```python
from build123d import *

# Parameters (mm, degrees)
BOSS_EXTRUDE4_DEPTH = 20
SKETCH6_R           = 1.75
CUT_EXTRUDE3_DEPTH  = 51.482948977
SKETCH7_R           = 3.3782
CUT_EXTRUDE4_DEPTH  = 52.051285634
SKETCH8_W           = 5.5
SKETCH8_H           = 5
BOSS_EXTRUDE5_DEPTH = 5


with BuildPart() as part:
    # Sketch5 → Boss-Extrude4 (new body)
    with BuildSketch(Plane(origin=(0, 0, 0), x_dir=(0, 0, -1), z_dir=(1, 0, 0))):
        Polygon((0, 0), (0, 20), (-21.213203436, 41.213203436), (-25.213203436, 41.213203436), (-4, 20), (-4, 0), align=None)
    extrude(amount=BOSS_EXTRUDE4_DEPTH)

    # Sketch6 → Cut-Extrude3 (cut, through all)
    with BuildSketch(Plane.XY.offset(4)):
        with Locations((10, 10)):
            Circle(SKETCH6_R)
    extrude(amount=-CUT_EXTRUDE3_DEPTH, mode=Mode.SUBTRACT)

    # Sketch7 → Cut-Extrude4 (cut, through all)
    with BuildSketch(Plane(origin=(0, 8, -8), x_dir=(1, 0, 0), z_dir=(0, -0.7071067811865489, 0.7071067811865462))):
        with Locations(Location((10, 31.970562748, 0), (0, 0, 270))):
            Circle(SKETCH7_R)
    extrude(amount=-CUT_EXTRUDE4_DEPTH, mode=Mode.SUBTRACT)

    # Sketch8 → Boss-Extrude5 (add)
    with BuildSketch(Plane(origin=(0, 0, 0), x_dir=(-1, 0, 0), z_dir=(0, 0, -1))):
        with Locations((-10, 17.5)):
            Rectangle(SKETCH8_W, SKETCH8_H)
        with Locations((-10, 2.5)):
            Rectangle(SKETCH8_W, SKETCH8_H)
    extrude(amount=BOSS_EXTRUDE5_DEPTH)


solid = part.part
```
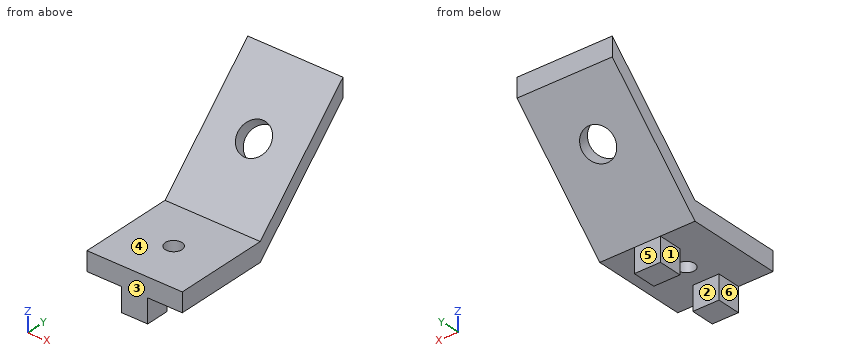
Geometry check sheet. Reference: the model listing, model coordinates, mm. Face numbers are marked on the shaded views. A direction names the side the tool comes from. Coordinates: 2 decimals unless noted, no trailing zeros. Order: outer loops, then holes, each group sorted by start corner. A loop starts at its lowest first (then second) coordinate and runs counter-clockwise, first axis right, second up.
Q1. Sectioned sample at B-B on x = 10. Record the cut outline in (y, z).
Reply:
outline: (0, -5) - (5, -5) - (5, 0) - (8.25, 0) - (8.25, 4) - (0, 4) - close; (11.75, 0) - (15, 0) - (15, -5) - (20, -5) - (20, 0) - (30.22, 10.22) - (28.22, 12.22) - (20, 4) - (11.75, 4) - close; (33, 17) - (35, 15) - (41.21, 21.21) - (41.21, 25.21) - close
Q2. Thickness scan on probe 1 along Y at (x, z) = (10, 1.1); probe 2 along Y at (x, z) = (10, 2.4); probe 3 along Z at (x, y) = (16.5, 12). Record the ranges inside material, lowest first.
Reply:
probe 1: y = 0 to 8.25, 11.75 to 21.1
probe 2: y = 0 to 8.25, 11.75 to 22.4
probe 3: z = 0 to 4
Q3. Sectioned sample at A-A on y = 10. Record the cut outline in (x, z).
Reply:
outline: (0, 0) - (8.25, 0) - (8.25, 4) - (0, 4) - close; (11.75, 0) - (20, 0) - (20, 4) - (11.75, 4) - close
Q4. Depth check by flat-ended pin: pin 1 Ø3 at (x, z) = (14, 15) entering from +Y; pin 2 Ø1 at (x, z) = (5, 13.5) entering from +Y; pin 3 Ø10 at (x, y) = (10.5, 12.5) entering from +Z. Enter the tip coordinate at first touch or a pass-through.
Reply:
pin 1: stops at y = 36.5
pin 2: stops at y = 34
pin 3: stops at z = 4
Q5. Tool access check on the marked faces 4, 5 and 6. Record the directions out of +Z, -Z, +X, -X, +Y, -Y that give a thin tool (end or side, any length) a straight path to the whole face; none if there is none.
Reply:
face 4: +Z, +X, -X, -Y
face 5: -Z, +X, -X, +Y
face 6: -Z, -X, +Y, -Y
Q6. Sectioned sample at C-C on y = 15.5. Record the cut outline in (x, z).
Reply:
outline: (0, 0) - (7.25, 0) - (7.25, -5) - (12.75, -5) - (12.75, 0) - (20, 0) - (20, 4) - (0, 4) - close
Q7. Sectioned sample at D-D on x = 3. Record the cut outline in (y, z), and give its area (3 significant figures).
Reply:
outline: (0, 0) - (20, 0) - (41.21, 21.21) - (41.21, 25.21) - (20, 4) - (0, 4) - close
area: 165 mm2
Q8. Draft check along Y on the marked faces 1, 2 and 3. Enter one of: released by +Y, released by -Y, zero draft, split by the parting line, or undercut.
Reply:
face 1: zero draft
face 2: undercut
face 3: released by -Y
